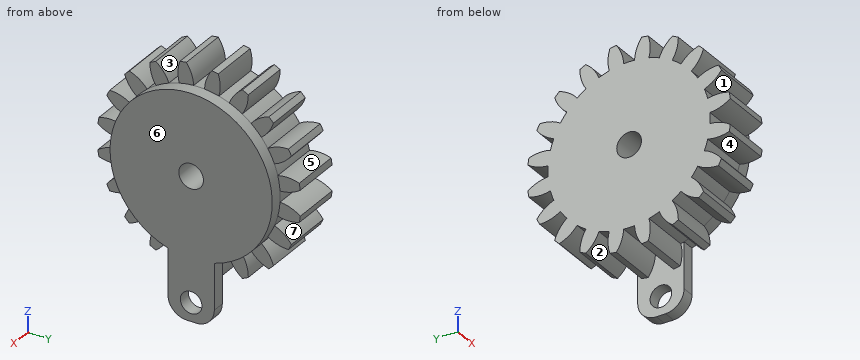
```python
from build123d import *

# Parameters (mm, degrees)
BASPROSKE_W         = 8
BASPROSKE_H         = 16.5
TOOTHCUT_DEPTH      = 25.667792767
TEETHCUTS_COUNT     = 20
TEETHCUTS_ANGLE     = 342
BORSKE_R            = 2
BORE_DEPTH          = 50.0000508
SKETCH1_R           = 1.75
BOSS_EXTRUDE1_DEPTH = 2
BOSS_EXTRUDE2_DEPTH = 2
SKETCH3_R           = 2
CUT_EXTRUDE1_DEPTH  = 15
FILLET1_R           = 3


with BuildPart() as part:
    # BasProSke → Base-Revolve (revolve)
    with BuildSketch(Plane(origin=(0, 0, 0), x_dir=(1, 0, 0), z_dir=(0, 1, 0)), mode=Mode.PRIVATE) as base_revolve_sk:
        with Locations((4, 8.25)):
            Rectangle(BASPROSKE_W, BASPROSKE_H)
    revolve(base_revolve_sk.sketch.rotate(Axis((-10, 0, 0), (1, 0, 0)), 180), axis=Axis((-10, 0, 0), (1, 0, 0)))

    # TooCutSke → ToothCut (cut, through all)
    with BuildSketch(Plane(origin=(0, 0, 0), x_dir=(0, 0, -1), z_dir=(1, 0, 0))):
        with BuildLine():
            ThreePointArc((0.877929023, 13.094602576), (0, 13.124), (-0.877929023, 13.094602576))
            ThreePointArc((-0.877929023, 13.094602576), (-1.227785764, 14.834041313), (-2.071065599, 16.395106966))
            ThreePointArc((-2.071065599, 16.395106966), (0, 16.5254), (2.071065599, 16.395106966))
            ThreePointArc((2.071065599, 16.395106966), (1.227785764, 14.834041313), (0.877929023, 13.094602576))
        make_face()
    toothcut = extrude(amount=TOOTHCUT_DEPTH, mode=Mode.SUBTRACT)

    # TeethCuts: ToothCut ×20 about axis
    teethcuts_axis = Axis((-10, 0, 0), (1, 0, 0))
    for i in range(1, TEETHCUTS_COUNT):
        add(toothcut.rotate(teethcuts_axis, i * TEETHCUTS_ANGLE / (TEETHCUTS_COUNT - 1)), mode=Mode.SUBTRACT)

    # BorSke → Bore (cut, symmetric)
    with BuildSketch(Plane(origin=(0, 0, 0), x_dir=(0, 0, -1), z_dir=(1, 0, 0))):
        with Locations(Location((0, 0, 0), (0, 0, 180))):
            Circle(BORSKE_R)
    extrude(amount=BORE_DEPTH, both=True, mode=Mode.SUBTRACT)

    # Sketch1 → Boss-Extrude1 (add)
    with BuildSketch(Plane(origin=(8, 0, 0), x_dir=(0, 0, -1), z_dir=(1, 0, 0))):
        Polygon((0, 0), (0, 3.75), (20, 3.75), (23, 3.75), (23, -3.75), (0, -3.75), align=None)
        with Locations((20, 0)):
            Circle(SKETCH1_R, mode=Mode.SUBTRACT)
    extrude(amount=BOSS_EXTRUDE1_DEPTH)

    # Sketch2 → Boss-Extrude2 (add)
    with BuildSketch(Plane(origin=(8, 0, 0), x_dir=(0, 0, -1), z_dir=(1, 0, 0))):
        with BuildLine():
            Line((0, 3.75), (12.576838872, 3.75))
            ThreePointArc((12.576838872, 3.75), (-13.124, 0), (12.576838872, -3.75))
            Line((12.576838872, -3.75), (0, -3.75))
            Line((0, -3.75), (0, 3.75))
        make_face()
    extrude(amount=BOSS_EXTRUDE2_DEPTH)

    # Sketch3 → Cut-Extrude1 (cut)
    with BuildSketch(Plane.ZY):
        Circle(SKETCH3_R)
    extrude(amount=-CUT_EXTRUDE1_DEPTH, mode=Mode.SUBTRACT)

    # Fillet1
    fillet1_edges = [part.edges().sort_by_distance(p)[0] for p in [
        (9, -3.75, -23),
        (9, 3.75, -23),
    ]]
    fillet(fillet1_edges, radius=FILLET1_R)


solid = part.part
```
Could you check a few things on this model? Use its own coordinates, in mm. Face numbers are marked on the shaded views. A direction names the side the tool comes from. Coordinates: 2 decimals unless noted, no trailing zeros. Loops run counter-clockwise (first coordinate to the right, second up) from the corner with the lowest first, then second, coordinate; pieces in that order, holes last. Notation, with made-up numbers: M 66,19 L 92,19 A21 cw 92,24 Z; hole C 18,52 d2. An arc over 180 degrees is marked long. Put each result on its own line as item: value. Start each with the question number.
(1) Suppose I cut it at C-C on x = 9. Please give me the cut outline in (y, z), then the cut area to 3 significant figures.
(2) Suppose I cut it at A-A on z = 0. Please give me the cut outline in (x, y), then the cut area to 3 significant figures.
(3) Suppose I cut it at D-D on z = 7.5. Please give me the cut outline in (x, y).
(4) I need wall thicknesses on line 1 (Z direction, x = 4.25, y = -14.5); line 2 (Z direction, x = 4, y = -13); line 3 (Y direction, x = 8.65, z = -20). Which ranges of each line are inside material? Lowest first, please. Write a range as from..to.
(5) For the marked faces 1, 2, 3 and 4, which set-ups out of +Z, -Z, +X, -X, +Y, -Y let a thin tool reach every point of the face, with its end or its side?
(6) Thinking about a two-plate mould opening in Y: for the marked faces 5, 6 and 7, which applies, pulls with the +Y half, pulls with the -Y half, needs draft (parallel to the pull), parting line crosses it, or undercut?
(7) Suppose I cut it at B-B on y = 0. Please give me the cut outline in (x, z).
(8) Will these pins go through, and if not, where does the flat tip stop? P1, Ø1, axis at x = 6, y = 10.5, coming from the -Z side; P2, Ø1.5, axis at x = 7, z = 3, coming from the +Y side; P3, Ø0.8, axis at y = -14.5, z = -2, coming from the +X side.
Solutions:
1. outline: M -3.75,-20 A3 ccw -0.75,-23 L 0.75,-23 A3 ccw 3.75,-20 L 3.75,-12.58 A13.12 ccw long -3.75,-12.58 Z; hole C 0,0 d4; hole C 0,-20 d3.5
1. area: 590 mm2
2. outline: M 0,-13.12 L 10,-13.12 L 10,-2 L 0,-2 Z; M 0,2 L 10,2 L 10,13.12 L 0,13.12 Z
2. area: 222 mm2
3. outline: M 0,-14.7 L 8,-14.7 L 8,-12.08 L 0,-12.08 Z; M 0,-10.77 L 10,-10.77 L 10,10.77 L 0,10.77 Z; M 0,12.08 L 8,12.08 L 8,14.7 L 0,14.7 Z
4. line 1: z = -7.87..-6.47, -3.42..-1.12, 1.12..3.42, 6.47..7.87
4. line 2: z = -7.8..-5.27, -3.28..3.28, 5.27..7.8
4. line 3: y = -3.75..-1.75, 1.75..3.75
5. face 1: +X, -X, -Y
5. face 2: -Z, +X, -X
5. face 3: +Z, +X, -X
5. face 4: +X, -X
6. face 5: undercut
6. face 6: needs draft
6. face 7: pulls with the +Y half
7. outline: M 0,-13.12 L 8,-13.12 L 8,-18.25 L 10,-18.25 L 10,-2 L 0,-2 Z; M 0,2 L 10,2 L 10,13.12 L 0,13.12 Z; M 8,-23 L 10,-23 L 10,-21.75 L 8,-21.75 Z
8. P1: stops at z = -11.94
8. P2: stops at y = 16.35
8. P3: stops at x = 8
